For this review, take the finished solid that the model builds, in its own axes (mm). A direction names the side the tool comes from. Coordinates: 2 decimals unless noted, no trailing zeros. Loops run counter-clockwise (first coordinate to the right, second up) from the corner with the lowest first, then second, coordinate; pieces in that order, holes last. Notation, with made-up numbers: (48, 2) - (79, 2) arc R19 ccw to (79, 16) - close; hole circle Ø1 at (84.25, 6.25). An arc over 180 degrees is marked (long way). Answer as a JSON object with one key per item and string values. Group by question number.
Item 1: To check wall thickness, follow line 1 (X direction, y = 10.5, z = 3.25); line 2 (Y direction, x = -32, z = 2); line 3 (Y direction, x = -27, z = 4.6). State the ranges of each line that lie inside material, in increasing order.
Item 2: Mouldability with a two-part tool opening along Y and no side actions: class faces 1 (the flat face through (23, 10, 2)), 2 (the flat face through (-37.5, 0, 2)), 3 (the cylindrical face through (36, 30.82, 2.54)) as released by +Y, released by -Y, zero draft, split by the parting line, or undercut.
Item 3: Tool access review of faces 4 (the flat face through (0, 32.25, 2)), 5 (the flat face through (-27, 2, 2)): name each direction out of +Z, -Z, +X, -X, +Y, -Y from which nothing blocks a thin tool from reaching the whole face with its end or side.
Item 4: We need section A-A (y = 6.5). Give the boundary of the cut face in (x, z).
Item 5: We need section C-C (z = 2.6). State how many separate pieces and enclosed holes the cut face has, then the cut area to 3 significant figures.
Item 6: We need section B-B (x = -28.5). Give the boundary of the cut face in (y, z), then the cut area to 4 significant figures.
from build123d import *

# Parameters (mm, degrees)
SKETCH_1_W           = 75
SKETCH_1_H           = 64.5
EXTRUDE_1_DEPTH      = 5
EXTRUDE_2_DEPTH      = 2
EXTRUDE_2_DEPTH_BACK = 2
SKETCH_4_R           = 2.5
CUT_EXTRUDE_2_DEPTH  = 60.516345229
SKETCH_5_W           = 8
SKETCH_5_H           = 16
CUT_EXTRUDE_3_DEPTH  = 60.516345229
FILLET_1_R           = 5
SKETCH_6_W           = 33.787770844
SKETCH_6_H           = 60.601542709
CUT_EXTRUDE_4_DEPTH  = 10


with BuildPart() as part:
    # 草圖1 → 填料-伸長1 (new body)
    with BuildSketch(Plane.XY):
        Rectangle(SKETCH_1_W, SKETCH_1_H)
    extrude(amount=EXTRUDE_1_DEPTH)

    # 草圖2 → 填料-伸長2 (add, two sides: drawn at the far end of the back side and taken through both)
    with BuildSketch(Plane(origin=(0, 0, 0), x_dir=(0, 0, -1), z_dir=(1, 0, 0)).offset(-EXTRUDE_2_DEPTH_BACK)):
        Polygon((0, 29.870222578), (0, 0), (0, -29.870222578), (33.104121336, -21), (33.104121336, 21), align=None)
    extrude(amount=EXTRUDE_2_DEPTH + EXTRUDE_2_DEPTH_BACK)

    # 草圖4 → 除料-伸長2 (cut, through all)
    with BuildSketch(Plane(origin=(0, 0, 0), x_dir=(-1, 0, 0), z_dir=(0, 0, -1))):
        with Locations((32, 26.75)):
            Circle(SKETCH_4_R)
        with Locations(Location((32, -26.75, 0), (0, 0, 180))):
            Circle(SKETCH_4_R)
        with Locations((-32, -26.75)):
            Circle(SKETCH_4_R)
        with Locations(Location((-32, 26.75, 0), (0, 0, 180))):
            Circle(SKETCH_4_R)
    extrude(amount=-CUT_EXTRUDE_2_DEPTH, mode=Mode.SUBTRACT)

    # 草圖5 → 除料-伸長3 (cut, through all)
    with BuildSketch(Plane(origin=(0, 0, 0), x_dir=(-1, 0, 0), z_dir=(0, 0, -1))):
        with Locations((-27, 10)):
            Rectangle(SKETCH_5_W, SKETCH_5_H)
        with Locations((27, 10)):
            Rectangle(SKETCH_5_W, SKETCH_5_H)
        with Locations((27, -10)):
            Rectangle(SKETCH_5_W, SKETCH_5_H)
        with Locations((-27, -10)):
            Rectangle(SKETCH_5_W, SKETCH_5_H)
    extrude(amount=-CUT_EXTRUDE_3_DEPTH, mode=Mode.SUBTRACT)

    # 圓角1
    fillet_1_edges = [part.edges().sort_by_distance(p)[0] for p in [
        (0, -21, -33.104121336),
        (0, 21, -33.104121336),
        (-37.5, 32.25, 2.5),
        (37.5, 32.25, 2.5),
        (37.5, -32.25, 2.5),
        (-37.5, -32.25, 2.5),
    ]]
    fillet(fillet_1_edges, radius=FILLET_1_R)

    # 草圖6 → 除料-伸長4 (cut)
    with BuildSketch(Plane(origin=(2, 0, 0), x_dir=(0, 0, -1), z_dir=(1, 0, 0))):
        with Locations((16.893885422, -0.430548776)):
            Rectangle(SKETCH_6_W, SKETCH_6_H)
    extrude(amount=-CUT_EXTRUDE_4_DEPTH, mode=Mode.SUBTRACT)


solid = part.part
Check sheet entries:
{
 "1": {"line 1": "x = -37.5 to -31, -23 to 23, 31 to 37.5", "line 2": "y = -32.25 to -29.25, -24.25 to 24.25, 29.25 to 32.25", "line 3": "y = -32.25 to -18, -2 to 2, 18 to 32.25"},
 "2": {"face 1": "undercut", "face 2": "zero draft", "face 3": "released by +Y"},
 "3": {"face 4": "+Z, -Z, +X, -X, +Y", "face 5": "+Z, -Z"},
 "4": {"outline": "(-37.5, 0) - (-31, 0) - (-31, 5) - (-37.5, 5) - close; (-23, 0) - (23, 0) - (23, 5) - (-23, 5) - close; (31, 0) - (37.5, 0) - (37.5, 5) - (31, 5) - close"},
 "5": {"separate pieces": "1", "enclosed holes": "8", "area": "4,230 mm2"},
 "6": {"outline": "(-32.25, 0) - (-18, 0) - (-18, 5) - (-32.25, 5) - close; (-2, 0) - (2, 0) - (2, 5) - (-2, 5) - close; (18, 0) - (32.25, 0) - (32.25, 5) - (18, 5) - close", "area": "162.5 mm2"}
}
